For this review, take the finished solid that the model builds, in its own axes (mm). A direction names the side the tool comes from. Round coordinates to 2 decimals unless told otherwise and drop trailing zeros. Write each loop counter-clockwise with the first axis right and the second up, starting at its lowest first coordinate (ties: lowest second). Pieces come first, ordered by that corner, then holes. Notation, with made-up numbers: (51, 27.5) -> (102, 27.5) arc R32 ccw to (102, 53.5) -> close; hole circle Ø4 at (28.5, 10). An arc over 180 degrees is marked (long way). Answer in a Markdown table with one row per item. Add a question column.
```python
from build123d import *

# Parameters (mm, degrees)
SKETCH003_W  = 43.15
SKETCH003_H  = 132.44
PAD_DEPTH    = 10
SKETCH004_W  = 29
SKETCH004_H  = 12.68
PAD001_DEPTH = 1
BINDER002_R  = 1.7
POCKET_DEPTH = 5


with BuildPart() as part:
    # Sketch003 → Pad (new body)
    with BuildSketch(Plane.XY):
        Rectangle(SKETCH003_W, SKETCH003_H)
    extrude(amount=PAD_DEPTH)

    # Sketch004 → Pad001 (join)
    with BuildSketch(Plane.XY):
        with Locations((0, 72.56)):
            Rectangle(SKETCH004_W, SKETCH004_H)
    pad001 = extrude(amount=PAD001_DEPTH)

    # Binder002 → Pocket (cut)
    with BuildSketch(Plane(origin=(-8.25, -72.5, 0), x_dir=(0, 1, 0), z_dir=(0, 0, 1))):
        Circle(BINDER002_R)
        with Locations((0, -16.5)):
            Circle(BINDER002_R)
        with Locations((145, 0)):
            Circle(BINDER002_R)
        with Locations((145, -16.5)):
            Circle(BINDER002_R)
    pocket = extrude(amount=POCKET_DEPTH, mode=Mode.SUBTRACT)

    # Mirrored: Pad001, Pocket across Sketch004 H_Axis
    add(pad001.mirror(Plane.ZX))
    add(pocket.mirror(Plane.ZX), mode=Mode.SUBTRACT)


solid = part.part
```
1. Clearance check with flat-ended pins moving along their axes: pin 1 Ø4 at (x, y) = (8.25, -72.5) entering from +Z; pin 2 Ø1 at (x, z) = (-14, 8.5) entering from -Y; pin 3 Ø0.8 at (y, z) = (-74.5, 0.5) entering from +X. State where each tip first meets the part, or that it passes through.
2. Tool access review of faces 5 (the flat face through (0, -73, 1)), 6 (the flat face through (0, 73, 1)), 7 (the cylindrical face through (-8.3, -70.8, 0.5)): name each direction out of +Z, -Z, +X, -X, +Y, -Y from which nothing blocks a thin tool from reaching the whole face with its end or side.
3. The part is to be moulded in two halves that separate along X. For faces 1 (the flat face through (21.575, -1, 5)), 2 (the flat face through (0, 1, 0)), 3 (the cylindrical face through (8.2, 70.8, 0.5)), 4 (the cylindrical face through (-8.3, 70.8, 0.5)), say which applies: pulls with the +X half, pulls with the -X half, needs draft (parallel to the pull), parting line crosses it, or undercut.
4. For L1, parallel to Y at x = 8.25, z = 0.4; L2, parallel to X at y = -72.5, z = 0.45; L3, parallel to Z at x = 9, y = 70.5, list the stretches that pass through material, from the lowest coordinate up. Write a range as [from, to].
5. We need section A-A (y = -72.5). Write out the cut boundary in (x, z), plus the area to 3 significant figures.
6. We need section B-B (x = 8.25). Write out the cut boundary in (y, z).
7. We need section C-C (x = -4). Write out the cut boundary in (y, z).
8. We need section D-D (z = 3.75). Write out the cut boundary in (x, y) (3 decimals), plus the area to 3 significant figures.
Response:
| question | item | result |
|---|---|---|
| 1 | pin 1 | z = 1 |
| 1 | pin 2 | y = -66.22 |
| 1 | pin 3 | x = 14.5 |
| 2 | face 5 | +Z, +X, -X, -Y |
| 2 | face 6 | +Z, +X, -X, +Y |
| 2 | face 7 | +Z, -Z |
| 3 | face 1 | pulls with the +X half |
| 3 | face 2 | needs draft |
| 3 | face 3 | undercut |
| 3 | face 4 | undercut |
| 4 | L1 | [-78.9, -74.2], [-70.8, 70.8], [74.2, 78.9] |
| 4 | L2 | [-14.5, -9.95], [-6.55, 6.55], [9.95, 14.5] |
| 4 | L3 | [0, 1] |
| 5 | outline | (-14.5, 0) -> (-9.95, 0) -> (-9.95, 1) -> (-14.5, 1) -> close; (-6.55, 0) -> (6.55, 0) -> (6.55, 1) -> (-6.55, 1) -> close; (9.95, 0) -> (14.5, 0) -> (14.5, 1) -> (9.95, 1) -> close |
| 5 | area | 22.2 mm2 |
| 6 | outline | (-78.9, 0) -> (-74.2, 0) -> (-74.2, 1) -> (-78.9, 1) -> close; (-70.8, 0) -> (70.8, 0) -> (70.8, 1) -> (66.22, 1) -> (66.22, 10) -> (-66.22, 10) -> (-66.22, 1) -> (-70.8, 1) -> close; (74.2, 0) -> (78.9, 0) -> (78.9, 1) -> (74.2, 1) -> close |
| 7 | outline | (-78.9, 0) -> (78.9, 0) -> (78.9, 1) -> (66.22, 1) -> (66.22, 10) -> (-66.22, 10) -> (-66.22, 1) -> (-78.9, 1) -> close |
| 8 | outline | (-21.575, -66.22) -> (21.575, -66.22) -> (21.575, 66.22) -> (-21.575, 66.22) -> close |
| 8 | area | 5,710 mm2 |
